from build123d import *

# Parameters (mm, degrees)
SKETCH2_R            = 10.3
BOSS_EXTRUDE1_DEPTH  = 39.5
CUT_EXTRUDE1_DEPTH   = 32.83
M7_CLEARANCE_HOLE1_D = 8


with BuildPart() as part:
    # Sketch2 → Boss-Extrude1 (new body)
    with BuildSketch(Plane.XY):
        with BuildLine():
            Line((-15.915, 0), (-15.915, -15.915))
            Line((-15.915, -15.915), (-15.915, -54.9))
            Line((-15.915, -54.9), (-12.515, -54.9))
            Line((-12.515, -54.9), (-12.515, -9.831683477))
            ThreePointArc((-12.515, -9.831683477), (0, -15.915), (12.515, -9.831683477))
            Line((12.515, -9.831683477), (12.515, -54.9))
            Line((12.515, -54.9), (15.915, -54.9))
            Line((15.915, -54.9), (15.915, -27.45))
            Line((15.915, -27.45), (15.915, 0))
            ThreePointArc((15.915, 0), (0, 15.915), (-15.915, 0))
        make_face()
        Circle(SKETCH2_R, mode=Mode.SUBTRACT)
    extrude(amount=BOSS_EXTRUDE1_DEPTH)

    # Sketch3 → Cut-Extrude1 (cut, through all)
    with BuildSketch(Plane.ZY.offset(15.915)):
        with BuildLine():
            ThreePointArc((19.75, -54.9), (12.873386553, -52.051613447), (10.025, -45.175))
            Line((10.025, -45.175), (0, -15.915))
            Line((0, -15.915), (0, -54.9))
            Line((0, -54.9), (19.75, -54.9))
        make_face()
        with BuildLine():
            Line((39.5, -15.915), (29.475, -45.175))
            ThreePointArc((29.475, -45.175), (26.626613447, -52.051613447), (19.75, -54.9))
            Line((19.75, -54.9), (39.5, -54.9))
            Line((39.5, -54.9), (39.5, -15.915))
        make_face()
    extrude(amount=-CUT_EXTRUDE1_DEPTH, mode=Mode.SUBTRACT)

    # M7 Clearance Hole1 (through all)
    with Locations(Plane.ZY.offset(15.915)):
        with Locations((19.75, -45.175), (19.75, -25.175)):
            Hole(M7_CLEARANCE_HOLE1_D / 2)


solid = part.part
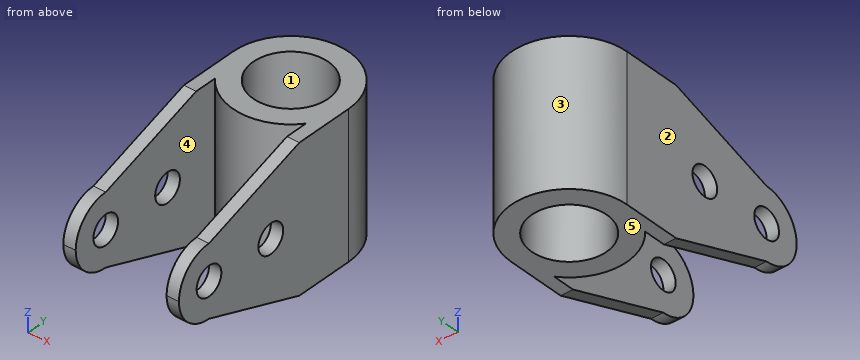
CAD build for the part. Positions are in the model's coordinates, mm. Face numbers are marked on the shaded views. A direction names the side the tool comes from. Coordinates: 2 decimals unless noted, no trailing zeros. Write each loop counter-clockwise with the first axis right and the second up, starting at its lowest first coordinate (ties: lowest second). Pieces come first, ordered by that corner, then holes. Notation, with made-up numbers: (37, -36) - (59, -36) arc R21 ccw to (59, -4) - close; hole circle Ø2 at (0.5, 42). An arc over 180 degrees is marked (long way). Use a Markdown table: item, result. Add a question column.
Item 1: Mould opens along Y. For the marked faces 1, 2 and 3 say: pulls with the +Y half, pulls with the -Y half, needs draft (parallel to the pull), parting line crosses it, or undercut.
Item 2: Band-saw the part on A-A, the plane x = 0. Give the cut face in (y, z) (3 decimals).
Item 3: Band-saw the part on D-D, the plane y = -31.5. Give the cut face in (x, z) (3 decimals), and give its area (3 significant figures).
Item 4: Band-saw the part on C-C, the plane z = 27.5. Give the cut face in (x, y) (3 decimals), and give its area (3 significant figures).
Item 5: Drill centre lines: L1, parallel to Y at x = -0.5, z = 31.5; L2, parallel to X at y = -47, z = 14 (3 decimals). Where is each one in solid material? Low to high. Write a range as from..to.
Item 6: Flat gauge pins, fed straight in: pin 1 (6 mm diameter, centred on x = 9, y = -47.5, fed in from -Z); pin 2 (8 mm diameter, centred on x = 3.5, z = 27, fed in from -Y) (3 decimals); pin 3 (4 mm diameter, centred on y = 6, z = 10, fed in from -X); pin 4 (10 mm diameter, centred on x = -10, y = -28.5, fed in from -Z). Where does each tip first touch, or does it go through?
Item 7: Band-saw the part on B-B, the plane y = -47.5. Give the cut face in (x, z) (3 decimals), and give its area (3 significant figures).
Item 8: 3-axis set-ups, long thin cutter, end or side, ignore diameter. For the marked faces 4 and 5: which of +Z, -Z, +X, -X, +Y, -Y reach the whole face in a straight line?
Numbers:
| question | item | result |
|---|---|---|
| 1 | face 1 | undercut |
| 1 | face 2 | needs draft |
| 1 | face 3 | pulls with the +Y half |
| 2 | outline | (-15.915, 0) - (-10.3, 0) - (-10.3, 39.5) - (-15.915, 39.5) - close; (10.3, 0) - (15.915, 0) - (15.915, 39.5) - (10.3, 39.5) - close |
| 3 | outline | (-15.915, 5.34) - (-12.515, 5.34) - (-12.515, 34.16) - (-15.915, 34.16) - close; (12.515, 5.34) - (15.915, 5.34) - (15.915, 34.16) - (12.515, 34.16) - close |
| 3 | area | 196 mm2 |
| 4 | outline | (-15.915, -51.05) - (-12.515, -51.05) - (-12.515, -9.832) arc R15.915 ccw to (12.515, -9.832) - (12.515, -51.05) - (15.915, -51.05) - (15.915, 0) arc R15.915 ccw to (-15.915, 0) - close; hole circle Ø20.6 at (0, 0) |
| 4 | area | 764 mm2 |
| 5 | L1 | -15.91..-10.29, 10.29..15.91 |
| 5 | L2 | -15.915..-12.515, 12.515..15.915 |
| 6 | pin 1 | through |
| 6 | pin 2 | y = -15.915 |
| 6 | pin 3 | x = -15.4 |
| 6 | pin 4 | z = 2.83 |
| 7 | outline | (-15.915, 10.307) - (-12.515, 10.307) - (-12.515, 16.495) - (-15.915, 16.495) - close; (-15.915, 23.005) - (-12.515, 23.005) - (-12.515, 29.193) - (-15.915, 29.193) - close; (12.515, 10.307) - (15.915, 10.307) - (15.915, 16.495) - (12.515, 16.495) - close; (12.515, 23.005) - (15.915, 23.005) - (15.915, 29.193) - (12.515, 29.193) - close |
| 7 | area | 84.2 mm2 |
| 8 | face 4 | +Z, -Z, -Y |
| 8 | face 5 | -Z, +X, -X, +Y, -Y |
